```python
from build123d import *

# Parameters (mm, degrees)
SKETCH1_W           = 100
SKETCH1_H           = 50
BOSS_EXTRUDE1_DEPTH = 3
FILLET1_R           = 5
SKETCH2_R           = 5
CUT_EXTRUDE1_DEPTH  = 3
SKETCH4_W           = 100
SKETCH4_H           = 2.5
CUT_EXTRUDE2_DEPTH  = 1


with BuildPart() as part:
    # Sketch1 → Boss-Extrude1 (new body)
    with BuildSketch(Plane(origin=(0, 0, 0), x_dir=(1, 0, 0), z_dir=(0, 1, 0))):
        Rectangle(SKETCH1_W, SKETCH1_H)
    extrude(amount=BOSS_EXTRUDE1_DEPTH)

    # Fillet1
    fillet1_edges = [part.edges().sort_by_distance(p)[0] for p in [
        (-50, 1.5, -25),
        (50, 1.5, -25),
        (50, 1.5, 25),
        (-50, 1.5, 25),
    ]]
    fillet(fillet1_edges, radius=FILLET1_R)

    # Sketch2 → Cut-Extrude1 (cut)
    with BuildSketch(Plane(origin=(0, 3, 0), x_dir=(1, 0, 0), z_dir=(0, 1, 0))):
        with Locations(Location((0, 0, 0), (0, 0, 270))):
            Circle(SKETCH2_R)
    extrude(amount=-CUT_EXTRUDE1_DEPTH, mode=Mode.SUBTRACT)

    # Sketch4 → Cut-Extrude2 (cut)
    with BuildSketch(Plane(origin=(0, 3, 0), x_dir=(1, 0, 0), z_dir=(0, 1, 0))):
        with Locations((0, 18.75)):
            Rectangle(SKETCH4_W, SKETCH4_H)
        with BuildLine():
            Line((-4.769696007, 1.5), (-50, 1.5))
            Line((-50, 1.5), (-50, -1))
            Line((-50, -1), (-4.898979486, -1))
            ThreePointArc((-4.898979486, -1), (-4.993327693, 0.258221909), (-4.769696007, 1.5))
        make_face()
        with BuildLine():
            Line((50, -1), (50, 1.5))
            Line((50, 1.5), (4.769696007, 1.5))
            ThreePointArc((4.769696007, 1.5), (4.942088629, 0.758788496), (5, 0))
            ThreePointArc((5, 0), (4.974680765, -0.50254481), (4.898979486, -1))
            Line((4.898979486, -1), (50, -1))
        make_face()
        with Locations((0, -18.25)):
            Rectangle(SKETCH4_W, SKETCH4_H)
    extrude(amount=-CUT_EXTRUDE2_DEPTH, mode=Mode.SUBTRACT)


solid = part.part
```
Work out the finished part from the listing and answer in its coordinate system (mm). A direction names the side the tool comes from. Give positions to 0.01 mm unless a question says otherwise; leave off trailing zeros. Order: outer loops, then holes, each group sorted by start corner. A loop starts at its lowest first (then second) coordinate and runs counter-clockwise, first axis right, second up. Notation, with made-up numbers: (-4.75, -37) -> (9.25, -37) arc R6 ccw to (9.25, -33) -> close; hole circle Ø9 at (16.5, 47.5). An arc over 180 degrees is marked (long way). Answer as CSV lines item,"result". Start each with the question number.
(1) Section C-C, the plane y = 1.15 is taken. Write down the section's boundary in (x, z), plus the area to 3 significant figures.
(2) Section A-A, the plane z = 0 is taken. Write down the section's boundary in (x, y), plus the area to 3 significant figures.
(3) For a pull along Z with two mould halves and no side action, classify faces 3 (the cylindrical face through (48, 2, 24)), 4 (the flat face through (-50, 1, 0)), 5 (the flat face through (-1, 2, 18)), 6 (the cylindrical face through (-1.915, 1.521, 4.619)) as released by +Z, released by -Z, zero draft, split by the parting line, or undercut.
(4) Which of the six approach directions +Z, -Z, +X, -X, +Y, -Y give full straight-line access (tool end or side, diameter ignored) to faces 1 (the flat face through (27, 2, 0)), 2 (the flat face through (-1, 0, -6))?
(5) Each of these flat-tipped pins is pushed along its axis until it touches: pin 1 Ø0.8 at (x, z) = (-24.5, 0) entering from +Y; pin 2 Ø3 at (x, z) = (-4, -18.5) entering from +Y. Where does it stop, or does it pass through?
(6) Section B-B, the plane x = 0 is taken. Write down the section's boundary in (y, z).
(7) Section D-D, the plane x = -27.5 is taken. Write down the section's boundary in (y, z).
(8) Consider line 1 along Z through (x, y) = (0, 2.35); line 2 along Z through (x, y) = (12.5, 2.5); line 3 along X through (y, z) = (1.4, 1). Determine where each line is inside the solid, lowest interval first.
Entries:
1,outline,"(-50, -20) arc R5 ccw to (-45, -25) -> (45, -25) arc R5 ccw to (50, -20) -> (50, 20) arc R5 ccw to (45, 25) -> (-45, 25) arc R5 ccw to (-50, 20) -> close; hole circle Ø10 at (0, 0)"
1,area,"4,900 mm²"
2,outline,"(-50, 0) -> (-5, 0) -> (-5, 2) -> (-50, 2) -> close; (5, 0) -> (50, 0) -> (50, 2) -> (5, 2) -> close"
2,area,"180 mm²"
3,face 3,"released by +Z"
3,face 4,"zero draft"
3,face 5,"undercut"
3,face 6,"undercut"
4,face 1,"+X, -X, +Y"
4,face 2,"+Z, -Z, +X, -X, -Y"
5,pin 1,"y = 2"
5,pin 2,"y = 3"
6,outline,"(0, -25) -> (3, -25) -> (3, -20) -> (2, -20) -> (2, -17.5) -> (3, -17.5) -> (3, -5) -> (0, -5) -> close; (0, 5) -> (3, 5) -> (3, 17) -> (2, 17) -> (2, 19.5) -> (3, 19.5) -> (3, 25) -> (0, 25) -> close"
7,outline,"(0, -25) -> (3, -25) -> (3, -20) -> (2, -20) -> (2, -17.5) -> (3, -17.5) -> (3, -1.5) -> (2, -1.5) -> (2, 1) -> (3, 1) -> (3, 17) -> (2, 17) -> (2, 19.5) -> (3, 19.5) -> (3, 25) -> (0, 25) -> close"
8,line 1,"-25 to -20, -17.5 to -5, 5 to 17, 19.5 to 25"
8,line 2,"-25 to -20, -17.5 to -1.5, 1 to 17, 19.5 to 25"
8,line 3,"-50 to -4.9, 4.9 to 50"
